Build history of the part. All positions in model axes, mm. Face numbers are marked on the shaded views. Round coordinates to 2 decimals unless told otherwise and drop trailing zeros. Write each loop counter-clockwise with the first axis right and the second up, starting at its lowest first coordinate (ties: lowest second). Pieces come first, ordered by that corner, then holes.
1) Saw through at A-A (z = -21.5). Write the cut outline in (x, y).
2) Saw through at D-D (x = 28). Write the cut outline in (y, z), plus the area to 3 significant figures.
3) Saw through at C-C (y = 4). Write the cut outline in (x, z), plus the area to 3 significant figures.
4) Wall check: probe 1 along X at (y, z) = (2.5, -24); probe 2 along Y at (x, z) = (24, -43.5); probe 3 along Z at (x, y) = (9.5, 4). Give the ranges that are in metal, low to high.
5) Flat gauge pins, fed straight in: pin 1 (2 mm diameter, centred on x = 4, z = -35.5, fed in from -Y); pin 2 (1.6 mm diameter, centred on x = -0.5, z = -21.5, fed in from +Y); pin 3 (1.3 mm diameter, centred on x = 14, y = 4.5, fed in from +Z); pin 4 (10 mm diameter, centred on x = 11.5, z = -43.5, fed in from +Y). Where does each tip first touch, or does it go through?
6) Pull direction X, two halves, no side cores. Call the marked faces 1, 2 and 3: +X half, -X half, draft (parallel to the pull), parting line (faces both ways), or undercut.
7) Saw through at B-B (y = 0.75). Write the cut outline in (x, z).
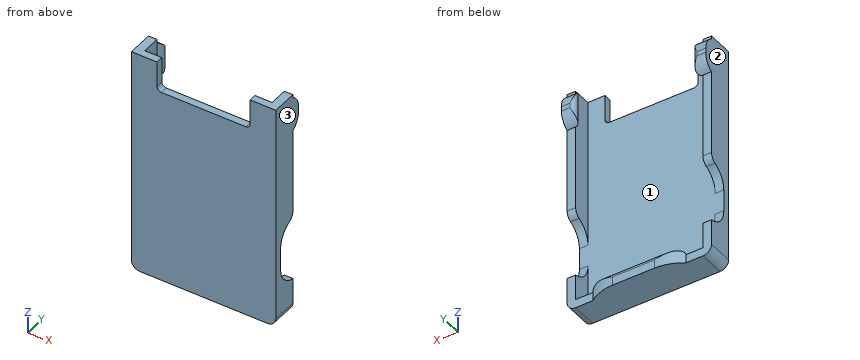
from build123d import *

# Parameters (mm, degrees)
SKETCH1_W               = 33.75000000000001
SKETCH1_H               = 55.99999999999999
SKETCH1_W_2             = 29.750000000000004
SKETCH1_H_2             = 52.00000000000001
BOSS_EXTRUDE1_DEPTH     = 6
BOSS_EXTRUDE2_DEPTH     = 1.7
SKETCH3_W               = 29.750000000000004
SKETCH3_H               = 4.3
CUT_EXTRUDE1_DEPTH      = 63.92902748334825
SKETCH5_W               = 21.750000000000004
SKETCH5_H               = 2.999999999999986
SKETCH5_W_2             = 2.9999999999999996
SKETCH5_H_2             = 8
BOSS_EXTRUDE3_DEPTH     = 2
CUT_EXTRUDE2_DEPTH      = 62.66137364671663
CUT_EXTRUDE2_DEPTH_BACK = 62.66137364671663
CUT_EXTRUDE3_DEPTH      = 62.66137364671663
CUT_EXTRUDE3_DEPTH_BACK = 62.66137364671663
CUT_EXTRUDE4_START      = -21.75
CUT_EXTRUDE4_DEPTH      = 21.75
FILLET1_R               = 10
FILLET2_R               = 4
CUT_EXTRUDE5_DEPTH      = 65.17992314238798
SKETCH12_W              = 21.750000000000004
SKETCH12_H              = 6.999999999999999
CUT_EXTRUDE6_DEPTH      = 63.958339642557306
FILLET4_R               = 2
FILLET5_R               = 1
CUT_EXTRUDE7_DEPTH      = 64.15110873264877
CUT_EXTRUDE7_DEPTH_BACK = 64.15110873264877
SKETCH13_W              = 14.999999999999996
SKETCH13_H              = 4.300000000000001
FILLET6_R               = 5
FILLET7_R               = 2


# Read off the part's stored shape, not the designer's step: Cut-Extrude4
with BuildPart() as part:
    # Sketch1 → Boss-Extrude1 (new body)
    with BuildSketch(Plane(origin=(0, 0, 0), x_dir=(1, 0, 0), z_dir=(0, 1, 0))):
        with Locations((14.875000000000002, 25.999999999999996)):
            Rectangle(SKETCH1_W, SKETCH1_H)
        with Locations((14.875000000000002, 26.000000000000004)):
            Rectangle(SKETCH1_W_2, SKETCH1_H_2, mode=Mode.SUBTRACT)
    extrude(amount=BOSS_EXTRUDE1_DEPTH)

    # Sketch2 → Boss-Extrude2 (add)
    with BuildSketch(Plane.XZ):
        Polygon((-1.9999999999999996, 2), (31.749999999999993, 2), (31.75, -53.99999999999999), (-1.9999999999999927, -53.99999999999999), align=None)
    extrude(amount=-BOSS_EXTRUDE2_DEPTH)

    # Sketch3 → Cut-Extrude1 (cut, through all)
    with BuildSketch(Plane(origin=(0, 0, 0), x_dir=(-1, 0, 0), z_dir=(0, 0, -1))):
        with Locations((-14.875000000000002, 3.85)):
            Rectangle(SKETCH3_W, SKETCH3_H)
    extrude(amount=-CUT_EXTRUDE1_DEPTH, mode=Mode.SUBTRACT)

    # Sketch5 → Boss-Extrude3 (add)
    with BuildSketch(Plane(origin=(0, 6, 0), x_dir=(1, 0, 0), z_dir=(0, 1, 0))):
        with Locations((14.875000000000002, 52.5)):
            Rectangle(SKETCH5_W, SKETCH5_H)
        with Locations((-0.4999999999999998, 5.75)):
            Rectangle(SKETCH5_W_2, SKETCH5_H_2)
        Polygon((31.750000000000014, 9.750000000000004), (28.75000000000001, 9.750000000000004), (28.750000000000014, 1.7500000000000033), (31.75000000000002, 1.750000000000004), align=None)
    extrude(amount=BOSS_EXTRUDE3_DEPTH)

    # Sketch6 → Cut-Extrude2 (cut, two sides: drawn at the far end of the back side and taken through both)
    with BuildSketch(Plane.XY.offset(-1.7499999999999998).offset(-CUT_EXTRUDE2_DEPTH_BACK)):
        with BuildLine():
            Line((1, 8), (0, 8))
            ThreePointArc((0, 8), (0.7071067811865474, 7.707106781186548), (1.0000000000000002, 7.000000000000001))
            Line((1, 7.000000000000001), (1, 8))
        make_face()
        with BuildLine():
            Line((1, 6), (1, 7.000000000000001))
            ThreePointArc((1.0000000000000002, 7.000000000000001), (0.7071067811865479, 6.292893218813453), (1.2e-16, 6))
            Line((0, 6), (1, 6))
        make_face()
    extrude(amount=CUT_EXTRUDE2_DEPTH + CUT_EXTRUDE2_DEPTH_BACK, mode=Mode.SUBTRACT)

    # Sketch7 → Cut-Extrude3 (cut, two sides: drawn at the far end of the back side and taken through both)
    with BuildSketch(Plane.XY.offset(-1.749999999999997).offset(-CUT_EXTRUDE3_DEPTH_BACK)):
        with BuildLine():
            Line((28.750000000000014, 6), (29.75, 6))
            ThreePointArc((29.75, 6), (29.042893218813454, 6.292893218813452), (28.75, 7))
            Line((28.750000000000014, 7), (28.750000000000014, 6))
        make_face()
        with BuildLine():
            Line((28.750000000000014, 8), (28.750000000000014, 7))
            ThreePointArc((28.75, 7), (29.042893218813454, 7.707106781186548), (29.75, 8))
            Line((29.75, 8), (28.750000000000014, 8))
        make_face()
    extrude(amount=CUT_EXTRUDE3_DEPTH + CUT_EXTRUDE3_DEPTH_BACK, mode=Mode.SUBTRACT)

    # Cut-Extrude4 outline → Cut-Extrude4 (cut)
    with BuildSketch(Plane.ZY.offset(-4).offset(CUT_EXTRUDE4_START)):
        with BuildLine():
            Line((-51, 6), (-51, 6.99))
            ThreePointArc((-51, 6.99), (-51.296387635, 6.289366479), (-51.99995, 5.999999999))
            Line((-51.99995, 5.999999999), (-51, 6))
        make_face()
        with BuildLine():
            ThreePointArc((-51.99995, 8.000000001), (-51.296387635, 7.710633521), (-51, 7.01))
            Line((-51, 7.01), (-51, 8))
            Line((-51, 8), (-51.99995, 8.000000001))
        make_face()
    extrude(amount=CUT_EXTRUDE4_DEPTH, mode=Mode.SUBTRACT)

    # Fillet1
    # the kernel refuses this fillet: 10 mm, written as the material it takes off along each edge
    with BuildSketch(Plane(origin=(4, 8, -36.99994999999842), x_dir=(1.1324e-13, -1, 0), z_dir=(0, 0, -1))) as fillet1_piece_1:
        with BuildLine():
            CenterArc((10.000000000000679, -5.999999999999498), FILLET1_R, 143.13010235415956, 36.86989764584689)
            Line((6.7946e-13, -6.000000000000631), (-0.19999999999931983, -6.000000000000653))
            Line((-0.19999999999931983, -6.000000000000653), (-0.1999999999999993, -2.265e-14))
            Line((-0.1999999999999993, -2.265e-14), (-2.265e-14, 0.20000000000000018))
            ThreePointArc((-2.265e-14, 0.20000000000000018), (1.0000000000001283, 0.20000000000011342), (1.8400000000002954, 0.11999999999998998))
            Line((1.8400000000002954, 0.11999999999998998), (2.000000000000303, 0))
        make_face()
    extrude(amount=32.00005000000314, mode=Mode.SUBTRACT)
    with BuildSketch(Plane(origin=(25.750000000000004, 8, -69.00000000000158), x_dir=(-1, 0, 0), z_dir=(0, 0, 1))) as fillet1_piece_2:
        with BuildLine():
            CenterArc((6.000000000000632, 10), FILLET1_R, 233.13010235415308, 36.86989764584689)
            Line((2.2737e-13, 2.0000000000003038), (-0.11999999999978073, 1.8400000000003098))
            ThreePointArc((-0.11999999999978073, 1.8400000000003098), (-0.1999999999999993, 1.0000000000001519), (-0.1999999999999993, 0))
            Line((-0.1999999999999993, 0), (0, -0.1999999999999993))
            Line((0, -0.1999999999999993), (6.000000000000632, -0.1999999999999993))
            Line((6.000000000000632, -0.1999999999999993), (6.000000000000632, 0))
        make_face()
    extrude(amount=32.00005000000316, mode=Mode.SUBTRACT)

    # Fillet2
    # the kernel refuses this fillet: 4 mm, written as the material it takes off along each edge
    with BuildSketch(Plane(origin=(8.66025403784487, 8, -9.75), x_dir=(0, -1, 7.283e-14), z_dir=(-1, 0, 0))) as fillet2_piece_1:
        with BuildLine():
            CenterArc((4.000000000000252, 3.4641016151376567), FILLET2_R, 179.99999999999582, 60.000000000001364)
            Line((2.5229e-13, 3.464101615137948), (-0.07999999999974777, 3.464101615137954))
            Line((-0.07999999999974777, 3.464101615137954), (-0.08000000000000007, 5.83e-15))
            Line((-0.08000000000000007, 5.83e-15), (-5.83e-15, -0.08000000000000007))
            ThreePointArc((-5.83e-15, -0.08000000000000007), (1.000000000000036, -0.0800000000000729), (1.9600000000000801, -0.06928203230275251))
            Line((1.9600000000000801, -0.06928203230275251), (2.0000000000000835, 0))
        make_face()
    extrude(amount=19.32050807568974, mode=Mode.SUBTRACT)
    with BuildSketch(Plane(origin=(-10.66025403784487, 8, -1.7499999999999998), x_dir=(0, -1, -7.25e-14), z_dir=(1, 0, 0))) as fillet2_piece_2:
        with BuildLine():
            CenterArc((4.000000000000251, 3.464101615137658), FILLET2_R, 179.99999999999585, 60.000000000001364)
            Line((2.5114e-13, 3.464101615137948), (-0.07999999999974894, 3.464101615137954))
            Line((-0.07999999999974894, 3.464101615137954), (-0.08000000000000007, 5.8e-15))
            Line((-0.08000000000000007, 5.8e-15), (-5.8e-15, -0.08000000000000007))
            ThreePointArc((-5.8e-15, -0.08000000000000007), (1.000000000000036, -0.08000000000007257), (1.9600000000000801, -0.06928203230275319))
            Line((1.9600000000000801, -0.06928203230275319), (2.0000000000000835, 0))
        make_face()
    extrude(amount=19.32050807568974, mode=Mode.SUBTRACT)
    with BuildSketch(Plane(origin=(40.41025403784491, 8, -9.750000000000004), x_dir=(0, -1, 7.55e-14), z_dir=(-1, 0, 0))) as fillet2_piece_3:
        with BuildLine():
            CenterArc((4.000000000000261, 3.464101615137654), FILLET2_R, 179.99999999999568, 60.00000000000142)
            Line((2.6152e-13, 3.464101615137956), (-0.07999999999973854, 3.464101615137962))
            Line((-0.07999999999973854, 3.464101615137962), (-0.08000000000000007, 6.04e-15))
            Line((-0.08000000000000007, 6.04e-15), (-6.04e-15, -0.08000000000000007))
            ThreePointArc((-6.04e-15, -0.08000000000000007), (1.0000000000000375, -0.08000000000007557), (1.9600000000000835, -0.0692820323027524))
            Line((1.9600000000000835, -0.0692820323027524), (2.000000000000087, 0))
        make_face()
    extrude(amount=19.320508075689798, mode=Mode.SUBTRACT)
    with BuildSketch(Plane(origin=(21.08974596215511, 8, -1.7500000000000018), x_dir=(-2.2e-16, 0, -1), z_dir=(1, 0, -2.2e-16))) as fillet2_piece_4:
        with BuildLine():
            CenterArc((3.464101615137956, -4), FILLET2_R, 90, 60.00000000000145)
            Line((1.5055e-13, -2.000000000000087), (-0.06928203230260555, -1.9600000000000888))
            ThreePointArc((-0.06928203230260555, -1.9600000000000888), (-0.0800000000000003, -1.0000000000000435), (-0.08000000000000007, 0))
            Line((-0.08000000000000007, 0), (0, 0.08000000000000007))
            Line((0, 0.08000000000000007), (3.464101615137956, 0.08000000000000007))
            Line((3.464101615137956, 0.08000000000000007), (3.464101615137956, 0))
        make_face()
    extrude(amount=19.320508075689798, mode=Mode.SUBTRACT)

    # Sketch11 → Cut-Extrude5 (cut, through all)
    with BuildSketch(Plane.ZY.offset(2.000000000000001)):
        Polygon((2, 6), (-1, 6), (-1.0000000000000009, 0), (2, 0), align=None)
    extrude(amount=-CUT_EXTRUDE5_DEPTH, mode=Mode.SUBTRACT)

    # Sketch12 → Cut-Extrude6 (cut, through all)
    with BuildSketch(Plane(origin=(0, 1.7, 0), x_dir=(1, 0, 0), z_dir=(0, 1, 0))):
        with Locations((14.875000000000002, 4.5)):
            Rectangle(SKETCH12_W, SKETCH12_H)
    extrude(amount=-CUT_EXTRUDE6_DEPTH, mode=Mode.SUBTRACT)

    # Fillet4
    fillet4_edges = [part.edges().sort_by_distance(p)[0] for p in [
        (-1.9999999999999987, 3, -53.99999999999999),
        (31.75, 3, -53.99999999999999),
    ]]
    fillet(fillet4_edges, radius=FILLET4_R)

    # Fillet5
    fillet5_edges = [part.edges().sort_by_distance(p)[0] for p in [
        (4, 0.85, -8),
        (25.75, 0.85, -8),
    ]]
    fillet(fillet5_edges, radius=FILLET5_R)

    # Sketch13 → Cut-Extrude7 (cut, two sides: drawn at the far end of the back side and taken through both)
    with BuildSketch(Plane(origin=(0, 0, 0), x_dir=(0, 0, -1), z_dir=(1, 0, 0)).offset(-CUT_EXTRUDE7_DEPTH_BACK)):
        with Locations((38.5, 3.8499999999999996)):
            Rectangle(SKETCH13_W, SKETCH13_H)
    extrude(amount=CUT_EXTRUDE7_DEPTH + CUT_EXTRUDE7_DEPTH_BACK, mode=Mode.SUBTRACT)

    # Fillet6
    # the kernel refuses this fillet: 5 mm, written as the material it adds along each edge
    with BuildSketch(Plane(origin=(31.75, 1.7, -46), x_dir=(0, 4e-17, 1), z_dir=(-1, 0, 0)), Plane(origin=(0, 1.7, -46), x_dir=(0, 4e-17, 1), z_dir=(-1, 0, 0))) as fillet6_piece_1:
        with BuildLine():
            CenterArc((4.9507575177946705, 5), FILLET6_R, 188.04784624731144, 81.95215375268856)
            Line((4.283e-14, 4.300000000000006), (-0.09901515035584632, 4.286000000000006))
            ThreePointArc((-0.09901515035584632, 4.286000000000006), (-0.10000000000000132, 2.150000000000003), (-0.10000000000000142, 0))
            Line((-0.10000000000000142, 0), (0, -0.10000000000000009))
            Line((0, -0.10000000000000009), (4.9507575177946705, -0.10000000000000009))
            Line((4.9507575177946705, -0.10000000000000009), (4.9507575177946705, 0))
        make_face()
    extrude(amount=2)
    with BuildSketch(Plane(origin=(29.75, 1.7, -31), x_dir=(0, 4e-17, -1), z_dir=(1, 0, 0)), Plane(origin=(-2, 1.7, -31), x_dir=(0, 4e-17, -1), z_dir=(1, 0, 0))) as fillet6_piece_2:
        with BuildLine():
            CenterArc((4.9507575177946705, 5), FILLET6_R, 188.04784624731144, 81.95215375268856)
            Line((4.283e-14, 4.300000000000006), (-0.09901515035584987, 4.286000000000006))
            ThreePointArc((-0.09901515035584987, 4.286000000000006), (-0.10000000000000132, 2.150000000000003), (-0.10000000000000142, 0))
            Line((-0.10000000000000142, 0), (0, -0.10000000000000009))
            Line((0, -0.10000000000000009), (4.9507575177946705, -0.10000000000000009))
            Line((4.9507575177946705, -0.10000000000000009), (4.9507575177946705, 0))
        make_face()
    extrude(amount=2)

    # Fillet7
    fillet7_edges = [part.edges().sort_by_distance(p)[0] for p in [
        (-1, 6, -31),
        (30.75, 6, -31),
    ]]
    fillet(fillet7_edges, radius=FILLET7_R)


solid = part.part
Evaluation:
1. outline: (-2, 0) - (31.75, 0) - (31.75, 6) - (29.75, 6) - (29.75, 1.7) - (0, 1.7) - (0, 6) - (-2, 6) - close
2. outline: (0, -54) - (6, -54) - (6, -52) - (1.7, -52) - (1.7, -1) - (0, -1) - close
2. area: 98.7 mm2
3. outline: (-2, -52) arc R2 ccw to (0, -54) - (29.75, -54) arc R2 ccw to (31.75, -52) - (31.75, -45.26) - (29.75, -45.26) - (29.75, -52) - (0, -52) - (0, -45.26) - (-2, -45.26) - close; (-2, -31.74) - (0, -31.74) - (0, -1) - (-2, -1) - close; (29.75, -31.74) - (31.75, -31.74) - (31.75, -1) - (29.75, -1) - close
3. area: 216 mm2
4. probe 1: x = -2 to 0, 29.75 to 31.75
4. probe 2: y = 0 to 1.7
4. probe 3: z = -54 to -52
5. pin 1: stops at y = 0
5. pin 2: stops at y = 6
5. pin 3: stops at z = -52
5. pin 4: stops at y = 1.7
6. face 1: undercut
6. face 2: -X half
6. face 3: +X half
7. outline: (-2, -52) arc R2 ccw to (0, -54) - (29.75, -54) arc R2 ccw to (31.75, -52) - (31.75, -1) - (25.75, -1) - (25.75, -7) arc R1 cw to (24.75, -8) - (5, -8) arc R1 cw to (4, -7) - (4, -1) - (-2, -1) - close
